```python
from build123d import *

# Parameters (mm, degrees)
PAD_DEPTH       = 3
SKETCH001_R     = 2.125
POCKET_DEPTH    = 2.15
CHAMFER_SIZE    = 0.2
CHAMFER001_SIZE = 0.2


with BuildPart() as part:
    # Sketch → Pad (new body)
    with BuildSketch(Plane.XY):
        Polygon((2.309401, 4), (-2.309401, 4), (-4.618802, 0), (-2.309401, -4), (2.309401, -4), (4.618802, -8), (9.237604, -8), (11.547005, -4), (9.237604, 0), (11.547005, 4), (9.237604, 8), (4.618802, 8), align=None)
    extrude(amount=PAD_DEPTH)

    # Sketch001 → Pocket (cut)
    with BuildSketch(Plane.XY):
        Circle(SKETCH001_R)
    extrude(amount=POCKET_DEPTH, mode=Mode.SUBTRACT)

    # Chamfer
    chamfer_edges = [part.edges().sort_by_distance(p)[0] for p in [
        (0, 4, 3),
        (-3.464102, 2, 3),
        (-3.464102, -2, 3),
        (0, -4, 3),
        (3.464102, -6, 3),
        (6.928203, -8, 3),
        (10.392305, -6, 3),
        (10.392305, -2, 3),
        (10.392305, 2, 3),
        (10.392305, 6, 3),
        (6.928203, 8, 3),
        (3.464102, 6, 3),
    ]]
    chamfer(chamfer_edges, length=CHAMFER_SIZE)

    # Chamfer001
    chamfer001_edges = [part.edges().sort_by_distance(p)[0] for p in [
        (0, 4, 0),
        (3.464102, 6, 0),
        (-3.464102, 2, 0),
        (6.928203, 8, 0),
        (-3.464102, -2, 0),
        (10.392305, 6, 0),
        (0, -4, 0),
        (10.392305, 2, 0),
        (3.464102, -6, 0),
        (10.392305, -2, 0),
        (6.928203, -8, 0),
        (10.392305, -6, 0),
        (-2.125, 0, 0),
    ]]
    chamfer(chamfer001_edges, length=CHAMFER001_SIZE)


solid = part.part
```
The listing builds one solid part. Answer for the finished solid, in the listing's coordinates (mm). A direction names the side the tool comes from. Round coordinates to 2 decimals unless told otherwise and drop trailing zeros. Write each loop counter-clockwise with the first axis right and the second up, starting at its lowest first coordinate (ties: lowest second). Pieces come first, ordered by that corner, then holes. Notation, with made-up numbers: (-30, -11.75) -> (19, -11.75) arc R23 cw to (19, 0.25) -> close; hole circle Ø9 at (-16.75, -20.75). An arc over 180 degrees is marked (long way). Answer as a JSON object with one key per item and string values. Group by question number.
Q1. Section D-D (y = 3.25) is taken. Write down the section's boundary in (x, z).
Q2. Section C-C (x = 10.25) is taken. Write down the section's boundary in (y, z).
Q3. Straight lines are drawn through the part: line 1 along Y through (x, z) = (0, 0.75) (3 decimals); line 2 along X through (y, z) = (-1.75, 0.7); line 3 along Z through (x, y) = (-0.5, 1.75). For each, find the intervals that lie inside material, in ascending order.
Q4. Section A-A (z = 1.7) is taken. Write down the section's boundary in (x, y) (3 decimals).
Q5. Determine the mould class of faces 3 (the face through (-3.448, 2.028, 1.482)), 4 (the face through (1.142, 1.792, 1.161)), 5 (the face through (10.41, -2.03, 1.48)), 6 (the face through (10.376, -6.028, 1.482)) for opening direction Y: pulls with the +Y half, pulls with the -Y half, needs draft (parallel to the pull), parting line crosses it, or undercut.
Q6. Section B-B (x = 0) is taken. Write down the section's boundary in (y, z) (3 decimals), plus the area to 3 significant figures.
Q7. Which of the six approach directions +Z, -Z, +X, -X, +Y, -Y give full straight-line access (tool end or side, diameter ignored) to faces 1 (the face through (0, 0, 2.15)), 2 (the face through (7, -8, 1))?
Q8. Each of these flat-tipped pins is pushed along its axis until it touches: pin 1 Ø1.5 at (x, z) = (0.5, 2) entering from +Y; pin 2 Ø0.8 at (x, z) = (1, 1.5) entering from -Y. Where does it stop, or does it pass through?
Check values:
{
 "1": {"outline": "(-2.74, 0.2) -> (-2.51, 0) -> (10.88, 0) -> (11.11, 0.2) -> (11.11, 2.8) -> (10.88, 3) -> (-2.51, 3) -> (-2.74, 2.8) -> close"},
 "2": {"outline": "(-6.25, 0.2) -> (-5.85, 0) -> (-2.15, 0) -> (-1.75, 0.2) -> (-1.75, 2.8) -> (-2.15, 3) -> (-5.85, 3) -> (-6.25, 2.8) -> close; (1.75, 0.2) -> (2.15, 0) -> (5.85, 0) -> (6.25, 0.2) -> (6.25, 2.8) -> (5.85, 3) -> (2.15, 3) -> (1.75, 2.8) -> close"},
 "3": {"line 1": "-4 to -2.125, 2.125 to 4", "line 2": "-3.61 to -1.21, 1.21 to 10.25", "line 3": "2.15 to 3"},
 "4": {"outline": "(-4.619, 0) -> (-2.309, -4) -> (2.309, -4) -> (4.619, -8) -> (9.238, -8) -> (11.547, -4) -> (9.238, 0) -> (11.547, 4) -> (9.238, 8) -> (4.619, 8) -> (2.309, 4) -> (-2.309, 4) -> close; hole circle Ø4.25 at (0, 0)"},
 "5": {"face 3": "pulls with the +Y half", "face 4": "undercut", "face 5": "undercut", "face 6": "pulls with the -Y half"},
 "6": {"outline": "(-4, 0.2) -> (-3.8, 0) -> (-2.325, 0) -> (-2.125, 0.2) -> (-2.125, 2.15) -> (2.125, 2.15) -> (2.125, 0.2) -> (2.325, 0) -> (3.8, 0) -> (4, 0.2) -> (4, 2.8) -> (3.8, 3) -> (-3.8, 3) -> (-4, 2.8) -> close", "area": "14.7 mm^2"},
 "7": {"face 1": "-Z", "face 2": "+Z, -Z, +X, -X, -Y"},
 "8": {"pin 1": "y = 4", "pin 2": "y = -4"}
}
